from build123d import *

# Parameters (mm, degrees)
SKETCH1_W           = 27.8
SKETCH1_H           = 33
SKETCH1_R           = 1.643134295
SKETCH1_R_2         = 3
SKETCH1_R_3         = 1.5
BOSS_EXTRUDE2_DEPTH = 3
SKETCH2_W           = 27.8
SKETCH2_H           = 3
BOSS_EXTRUDE4_DEPTH = 32
SKETCH4_R           = 1.5
CUT_EXTRUDE2_DEPTH  = 32


with BuildPart() as part:
    # Sketch1 → Boss-Extrude2 (new body)
    with BuildSketch(Plane(origin=(0, 0, 0), x_dir=(1, 0, 0), z_dir=(0, 1, 0))):
        with Locations((-63.812097694, -4.729298211)):
            Rectangle(SKETCH1_W, SKETCH1_H)
        with Locations(Location((-63.812097694, 7.770701789, 0), (0, 0, 270))):
            Circle(SKETCH1_R, mode=Mode.SUBTRACT)
        with Locations(Location((-63.812097694, -0.229298211, 0), (0, 0, 270))):
            Circle(SKETCH1_R_2, mode=Mode.SUBTRACT)
        with Locations(Location((-63.812097694, -8.229298211, 0), (0, 0, 270))):
            Circle(SKETCH1_R_3, mode=Mode.SUBTRACT)
        with Locations(Location((-73.312097694, -0.229298211, 0), (0, 0, 270))):
            Circle(SKETCH1_R_3, mode=Mode.SUBTRACT)
        with Locations(Location((-54.312097694, -0.229298211, 0), (0, 0, 270))):
            Circle(SKETCH1_R_3, mode=Mode.SUBTRACT)
    extrude(amount=BOSS_EXTRUDE2_DEPTH)

    # Sketch2 → Boss-Extrude4 (add)
    with BuildSketch(Plane(origin=(0, 3, 0), x_dir=(1, 0, 0), z_dir=(0, 1, 0))):
        with Locations((-63.812097694, -19.729298211)):
            Rectangle(SKETCH2_W, SKETCH2_H)
    extrude(amount=BOSS_EXTRUDE4_DEPTH)

    # Sketch4 → Cut-Extrude2 (cut)
    with BuildSketch(Plane(origin=(0, 0, 18.229298211), x_dir=(-1, 0, 0), z_dir=(0, 0, -1))):
        with Locations((53.912097694, 11)):
            Circle(SKETCH4_R)
        with Locations((73.712097694, 31)):
            Circle(SKETCH4_R)
        with Locations((53.912097694, 31)):
            Circle(SKETCH4_R)
        with Locations((73.712097694, 11)):
            Circle(SKETCH4_R)
    extrude(amount=-CUT_EXTRUDE2_DEPTH, mode=Mode.SUBTRACT)


solid = part.part
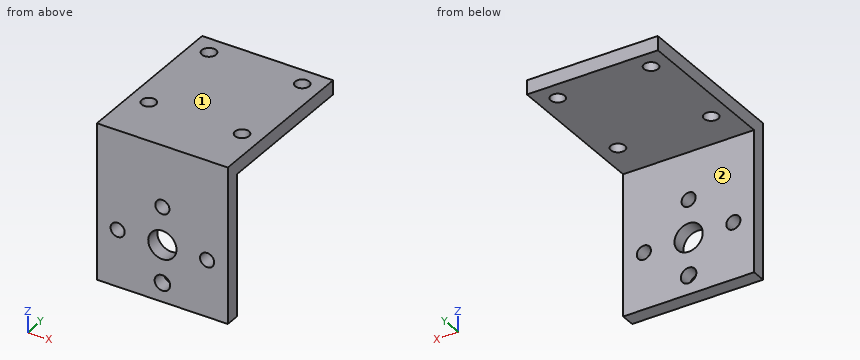
Could you check a few things on this model? Use its own coordinates, in mm. Face numbers are marked on the shaded views. A direction names the side the tool comes from. Coordinates: 2 decimals unless noted, no trailing zeros. Order: outer loops, then holes, each group sorted by start corner. A loop starts at its lowest first (then second) coordinate and runs counter-clockwise, first axis right, second up. Notation, with made-up numbers: (-28.75, 48) -> (-0.75, 48) arc R15 ccw to (-0.75, 59) -> close; hole circle Ø1 at (8, 71.25). An arc over 180 degrees is marked (long way). One line per question, with ' | ' between items.
Q1. Imagine slicing it at B-B on z = 0.5. Please give me the cut outline in (x, y), and give its area (3 significant figures).
Return value:
outline: (-77.71, 0) -> (-74.79, 0) -> (-74.79, 3) -> (-77.71, 3) -> close; (-71.84, 0) -> (-66.8, 0) -> (-66.8, 3) -> (-71.84, 3) -> close; (-60.82, 0) -> (-55.79, 0) -> (-55.79, 3) -> (-60.82, 3) -> close; (-52.84, 0) -> (-49.91, 0) -> (-49.91, 3) -> (-52.84, 3) -> close | area: 47.8 mm²
Q2. Imagine slicing it at C-C on x = -57.75. Please give me the cut outline in (y, z), and give its area (3 significant figures).
Return value:
outline: (0, -11.77) -> (3, -11.77) -> (3, 18.23) -> (35, 18.23) -> (35, 21.23) -> (0, 21.23) -> close | area: 195 mm²
Q3. I'm going to push flat-ended pins straight in: P1, Ø12, axis at x = -67, z = 8, coming from the +Y side; P2, Ø3.5, axis at x = -54.31, z = 0.23, coming from the -Y side. Where does each tip first touch, or does it pass through?
Return value:
P1: y = 3 | P2: y = 0
Q4. Imagine slicing it at D-D on y = 13. Please give me the cut outline in (x, z).
Return value:
outline: (-77.71, 18.23) -> (-49.91, 18.23) -> (-49.91, 21.23) -> (-77.71, 21.23) -> close
Q5. Imagine slicing it at A-A on y = 31. Please give me the cut outline in (x, z), and give its area (3 significant figures).
Return value:
outline: (-77.71, 18.23) -> (-75.21, 18.23) -> (-75.21, 21.23) -> (-77.71, 21.23) -> close; (-72.21, 18.23) -> (-55.41, 18.23) -> (-55.41, 21.23) -> (-72.21, 21.23) -> close; (-52.41, 18.23) -> (-49.91, 18.23) -> (-49.91, 21.23) -> (-52.41, 21.23) -> close | area: 65.4 mm²
Q6. On a 3-axis mill with a long thin cutter (end or side, diameter ignored), from which of +Z, -Z, +X, -X, +Y, -Y can I reach the whole of each face in a straight line? I mean the marked faces 1 and 2. Say none if no direction works.
Return value:
face 1: +Z, +X, -X, +Y, -Y | face 2: -Z, +X, -X, +Y
Q7. If I drill on L1, parallel to Y at x = -73.5, z = -4; L2, parallel to Z at x = -72, y = 27, over which ranges is the centre line in solid material (lowest first)?
Return value:
L1: 0 to 3 | L2: 18.23 to 21.23
